from build123d import *

# Parameters (mm, degrees)
SKETCH1_W             = 44
SKETCH1_H             = 44
SKETCH1_R             = 1.6
SKETCH1_R_2           = 1.75
SKETCH1_W_2           = 7.18
BOSS_EXTRUDE1_DEPTH   = 3.175
SKETCH2_W             = 10
SKETCH2_H             = 44
BOSS_EXTRUDE2_DEPTH   = 3.175
F_4_40_TAPPED_HOLE1_D = 2.2606
FILLET2_R             = 1.5875


with BuildPart() as part:
    # Sketch1 → Boss-Extrude1 (new body)
    # profile 1 of 2: a face of its own
    with BuildSketch(Plane(origin=(0, 0, 0), x_dir=(1, 0, 0), z_dir=(0, 1, 0))):
        with Locations((22, -22)):
            Rectangle(SKETCH1_W, SKETCH1_H)
        with Locations(Location((7, -37, 0), (0, 0, 270))):
            Circle(SKETCH1_R, mode=Mode.SUBTRACT)
        with Locations(Location((21.07, -28, 0), (0, 0, 270))):
            Circle(SKETCH1_R_2, mode=Mode.SUBTRACT)
        with Locations(Location((37, -37, 0), (0, 0, 270))):
            Circle(SKETCH1_R, mode=Mode.SUBTRACT)
        with Locations(Location((41.07, -28, 0), (0, 0, 270))):
            Circle(SKETCH1_R_2, mode=Mode.SUBTRACT)
        with Locations(Location((7, -7, 0), (0, 0, 270))):
            Circle(SKETCH1_R, mode=Mode.SUBTRACT)
        with Locations(Location((37, -7, 0), (0, 0, 270))):
            Circle(SKETCH1_R, mode=Mode.SUBTRACT)
    # profile 2 of 2: a face of its own
    with BuildSketch(Plane(origin=(0, 0, 0), x_dir=(1, 0, 0), z_dir=(0, 1, 0))):
        with Locations((47.59, -22)):
            Rectangle(SKETCH1_W_2, SKETCH1_H)
    extrude(amount=BOSS_EXTRUDE1_DEPTH)

    # Sketch2 → Boss-Extrude2 (add)
    with BuildSketch(Plane(origin=(0, 3.175, 0), x_dir=(1, 0, 0), z_dir=(0, 1, 0))):
        with Locations((-5, -22)):
            Rectangle(SKETCH2_W, SKETCH2_H)
        with Locations((56.18, -22)):
            Rectangle(SKETCH2_W, SKETCH2_H)
    extrude(amount=-BOSS_EXTRUDE2_DEPTH)

    # #4-40 Tapped Hole1 (through all)
    with Locations(Plane(origin=(-7, 3.175, 3), x_dir=(0, 0, 1), z_dir=(0, 1, 0))):
        with Locations((0, 0), (38, 0), (0, 65.18), (38, 65.18)):
            Hole(F_4_40_TAPPED_HOLE1_D / 2)

    # Fillet2
    fillet2_edges = [part.edges().sort_by_distance(p)[0] for p in [
        (-10, 1.5875, 0),
        (-10, 1.5875, 44),
        (61.18, 1.5875, 44),
        (61.18, 1.5875, 0),
    ]]
    fillet(fillet2_edges, radius=FILLET2_R)


solid = part.part
Read the model definition and answer for the solid it produces. Units are mm, in the model's axes. Give positions to 0.01 mm unless a question says otherwise; leave off trailing zeros. Write each loop counter-clockwise with the first axis right and the second up, starting at its lowest first coordinate (ties: lowest second). Pieces come first, ordered by that corner, then holes. Notation, with made-up numbers: (76, 35) -> (135, 35) arc R24 ccw to (135, 47) -> close; hole circle Ø2 at (-15, 56). An arc over 180 degrees is marked (long way). Answer as a JSON object with one key per item and string values. Group by question number.
1) Find section D-D (y = 1.55). Count the separate pieces of the cut face and the enclosed holes in it, and give its area (3 significant figures).
2) Find section C-C (x = -7). Write down the section's boundary in (y, z) (3 decimals), and give its area (3 significant figures).
3) Consider L1, parallel to X at y = 2.4, z = 7; L2, parallel to X at y = 1.85, z = 28; L3, parallel to X at y = 0.8, z = 42.5. Determine where each line is inside the solid, lowest interval first. Write a range as from..to.
4) This flat-tipped pin is pushed along its axis until it touches: P1, Ø4, axis at x = 37, z = 7, coming from the +Y side (3 decimals). Where does it stop, or does it pass through?
5) Find section B-B (z = 3). Write down the section's boundary in (x, y) (3 decimals).
6) The mould has two halves that part along Z. Classify faces 1 (the flat face through (25, 2, 0)), 2 (the flat face through (-10, 2, 22)), 3 (the cylindrical face through (-7.433, 1.565, 39.956)): +Z half, -Z half, draft (parallel to the pull), parting line (faces both ways), or undercut.
7) Find section A-A (x = 41.07). Write down the section's boundary in (y, z) (3 decimals), and give its area (3 significant figures).
Values follow:
{
 "1": {"separate pieces": "1", "enclosed holes": "10", "area": "3,060 mm2"},
 "2": {"outline": "(0, 0) -> (3.175, 0) -> (3.175, 1.87) -> (0, 1.87) -> close; (0, 4.13) -> (3.175, 4.13) -> (3.175, 39.87) -> (0, 39.87) -> close; (0, 42.13) -> (3.175, 42.13) -> (3.175, 44) -> (0, 44) -> close", "area": "125 mm2"},
 "3": {"L1": "x = -10..5.4, 8.6..35.4, 38.6..61.18", "L2": "x = -10..19.32, 22.82..39.32, 42.82..61.18", "L3": "x = -10..61.18"},
 "4": {"P1": "stops at y = 3.175"},
 "5": {"outline": "(-10, 0) -> (-8.13, 0) -> (-8.13, 3.175) -> (-10, 3.175) -> close; (-5.87, 0) -> (57.05, 0) -> (57.05, 3.175) -> (-5.87, 3.175) -> close; (59.31, 0) -> (61.18, 0) -> (61.18, 3.175) -> (59.31, 3.175) -> close"},
 "6": {"face 1": "-Z half", "face 2": "draft", "face 3": "undercut"},
 "7": {"outline": "(0, 0) -> (3.175, 0) -> (3.175, 26.25) -> (0, 26.25) -> close; (0, 29.75) -> (3.175, 29.75) -> (3.175, 44) -> (0, 44) -> close", "area": "129 mm2"}
}
